from build123d import *

# Parameters (mm, degrees)
F1_DEPTH  = 88
F2_R      = 1.778
F3_DEPTH  = 5
F4_R      = 1.778
F5_DEPTH  = 11.627384
F7_W      = 6.4
F7_H      = 21.920782
F8_DEPTH  = 25
F9_R      = 5
F10_DEPTH = 6
F11_W     = 2
F11_H     = 18
F12_DEPTH = 4


with BuildPart() as f1:
    # F0 (on Right) → F1 (new body)
    with BuildSketch(Plane.YZ):
        Polygon((0.151508, 14.999235), (0, 0), (18, 0), (18, 11), align=None)
    extrude(amount=F1_DEPTH)

    # F2 (on face) → F3 (cut)
    with BuildSketch(Plane(origin=(0, 3.207392, 14.314516), x_dir=(1, 0, 0), z_dir=(0, 0.218644, 0.975805))):
        with Locations((19.15, 2.659395)):
            Circle(F2_R)
        with Locations((12.95, 2.659395)):
            Circle(F2_R)
        with Locations((6.75, 2.659395)):
            Circle(F2_R)
        with Locations((15.65, 9.159395)):
            Circle(F2_R)
        with Locations((3.25, 9.159395)):
            Circle(F2_R)
        with Locations((75.05, 2.659395)):
            Circle(F2_R)
        with Locations((68.85, 2.659395)):
            Circle(F2_R)
        with Locations((81.25, 2.659395)):
            Circle(F2_R)
        with Locations((72.35, 9.159395)):
            Circle(F2_R)
        with Locations((78.55, 9.159395)):
            Circle(F2_R)
        with Locations((84.75, 9.159395)):
            Circle(F2_R)
        with Locations((9.45, 9.159395)):
            Circle(F2_R)
    extrude(amount=-F3_DEPTH, mode=Mode.SUBTRACT)

    # F4 (on face) → F5 (cut, through all)
    with BuildSketch(Plane(origin=(0, 0, 0), x_dir=(1, 0, 0), z_dir=(0, 0, -1))):
        with Locations((44, -15.2)):
            Circle(F4_R)
        with Locations((44, -2.8)):
            Circle(F4_R)
    extrude(amount=-F5_DEPTH, mode=Mode.SUBTRACT)

    # F7 (on offset) → F8 (cut)
    with BuildSketch(Plane.XY.offset(6)):
        with Locations((44, 7.695412)):
            Rectangle(F7_W, F7_H)
    extrude(amount=F8_DEPTH, mode=Mode.SUBTRACT)

    # F9 (on face) → F10 (cut)
    with BuildSketch(Plane(origin=(0, 0, 0), x_dir=(1, 0, 0), z_dir=(0, 0, -1))):
        with Locations((54, -12.2)):
            Circle(F9_R)
        with Locations((34, -12.2)):
            Circle(F9_R)
    extrude(amount=-F10_DEPTH, mode=Mode.SUBTRACT)

    # F11 (on face) → F12 (cut)
    with BuildSketch(Plane(origin=(0, 0, 0), x_dir=(1, 0, 0), z_dir=(0, 0, -1))):
        with Locations((87, -9)):
            Rectangle(F11_W, F11_H)
    extrude(amount=-F12_DEPTH, mode=Mode.SUBTRACT)


solid = f1.part
Could you check a few things on this model? Use its own coordinates, in mm. A direction names the side the tool comes from. Round coordinates to 2 decimals unless told otherwise and drop trailing zeros. Write each loop counter-clockwise with the first axis right and the second up, starting at its lowest first coordinate (ties: lowest second). Pieces come first, ordered by that corner, then holes. Notation, with made-up numbers: (87, 9) -> (112, 9) arc R12 ccw to (112, 20) -> close; hole circle Ø3 at (52.25, 78). An arc over 180 degrees is marked (long way). Use a Markdown table: item, result.
1. If we section it at B-B (z = 1.5): List the corners of the cut face in (x, y) for me, then the cut area to 3 significant figures.
Answer key:
| item | result |
|---|---|
| outline | (0, 0.02) -> (86, 0.02) -> (86, 18) -> (0, 18) -> close; hole circle Ø10 at (34, 12.2); hole circle Ø3.56 at (44, 2.8); hole circle Ø3.56 at (44, 15.2); hole circle Ø10 at (54, 12.2) |
| area | 1,370 mm^2 |
2. Please list where these lines run through material, in increasing order: probe 1 along Y at (x, z) = (44, 1.35); probe 2 along X at (y, z) = (12.2, 3.8); probe 3 along X at (y, z) = (12.2, 4.5).
Answer key:
| item | result |
|---|---|
| probe 1 | y = 0.01 to 1.02, 4.58 to 13.42, 16.98 to 18 |
| probe 2 | x = 0 to 29, 39 to 49, 59 to 86 |
| probe 3 | x = 0 to 29, 39 to 49, 59 to 88 |
3. Which directions (+Z, -Z, +X, -X, +Y, -Y) give clear straight access to the entire face, cutting with the end or side of a thin tool? Please do faces 5 (the face through (67.31, 9.2, 12.97)), 6 (the face through (81.23, 4.73, 8.85)).
Answer key:
| item | result |
|---|---|
| face 5 | +Z, +X, -X, +Y |
| face 6 | none |
4. If we section it at C-C (y = 15.2): List the corners of the cut face in (x, z) for me, then the cut area to 3 significant figures.
Answer key:
| item | result |
|---|---|
| outline | (0, 0) -> (30, 0) -> (30, 6) -> (38, 6) -> (38, 0) -> (42.22, 0) -> (42.22, 6) -> (40.8, 6) -> (40.8, 11.63) -> (0, 11.63) -> close; (45.78, 0) -> (50, 0) -> (50, 6) -> (58, 6) -> (58, 0) -> (86, 0) -> (86, 4) -> (88, 4) -> (88, 11.63) -> (47.2, 11.63) -> (47.2, 6) -> (45.78, 6) -> close |
| area | 862 mm^2 |
5. If we section it at A-A (x = 44): List the corners of the cut face in (y, z) for me.
Answer key:
| item | result |
|---|---|
| outline | (0, 0) -> (1.02, 0) -> (1.02, 6) -> (0.06, 6) -> close; (4.58, 0) -> (13.42, 0) -> (13.42, 6) -> (4.58, 6) -> close; (16.98, 0) -> (18, 0) -> (18, 6) -> (16.98, 6) -> close |
6. We'd pull the mould along Y, two halves only. Please class faces 1 (the face through (43, 18, 5)), 2 (the face through (44, 9, 6)), 3 (the face through (8.14, 12.78, 9.64)), 4 (the face through (45.642, 3.481, 2.958)): +Y half, -Y half, draft (parallel to the pull), parting line (faces both ways), or undercut.
Answer key:
| item | result |
|---|---|
| face 1 | +Y half |
| face 2 | draft |
| face 3 | undercut |
| face 4 | undercut |
7. For pin 1 Ø0.6 at (x, y) = (87, 6.5) entering from -Z; pin 2 Ø1 at (x, y) = (35, 7) entering from +Z; pin 3 Ø1.5 at (x, y) = (10.5, 4.5) entering from +Z; pin 4 Ø3 at (x, y) = (44, 15.2) entering from +Z, each with a flat end and sliding along its axis, tell me the tip position at first contact or that it passes through.
Answer key:
| item | result |
|---|---|
| pin 1 | stops at z = 4 |
| pin 2 | stops at z = 13.58 |
| pin 3 | stops at z = 14.19 |
| pin 4 | passes through |
8. If we section it at D-D (x = 54): List the corners of the cut face in (y, z) for me, then the cut area to 3 significant figures.
Answer key:
| item | result |
|---|---|
| outline | (0, 0) -> (7.2, 0) -> (7.2, 6) -> (17.2, 6) -> (17.2, 0) -> (18, 0) -> (18, 11) -> (0.15, 15) -> close |
| area | 173 mm^2 |
